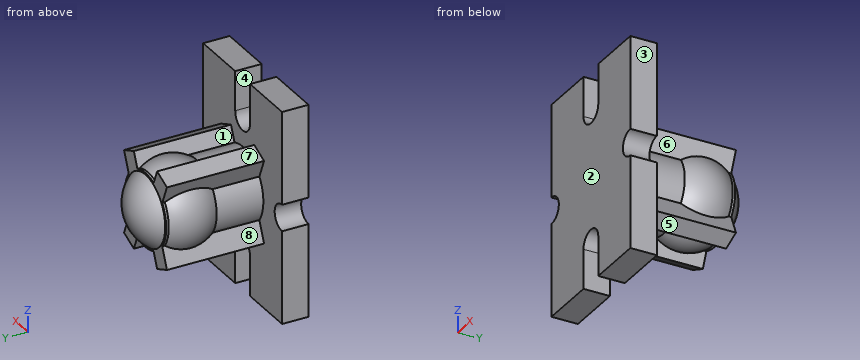
from build123d import *

# Parameters (mm, degrees)
EXTRUDE_1_DEPTH = 3
EXTRUDE_2_DEPTH = 11


with BuildPart() as part:
    # Sketch 1 → Extrude 1 (new body)
    with BuildSketch(Plane(origin=(0, 0, 0), x_dir=(1, 0, 0), z_dir=(0, 1, 0))):
        with BuildLine():
            Line((1.5, 12), (8, 12))
            Line((8, 12), (8, 1.5))
            ThreePointArc((8, 1.5), (6.5, 0), (8, -1.5))
            Line((8, -1.5), (8, -12))
            Line((8, -12), (1.5, -12))
            Line((1.5, -12), (1.5, -7.52))
            ThreePointArc((1.5, -7.52), (0, -6.02), (-1.5, -7.52))
            Line((-1.5, -7.52), (-1.5, -12))
            Line((-1.5, -12), (-8, -12))
            Line((-8, -12), (-8, -1.5))
            ThreePointArc((-8, -1.5), (-6.5, 0), (-8, 1.5))
            Line((-8, 1.5), (-8, 12))
            Line((-8, 12), (-1.5, 12))
            Line((-1.5, 12), (-1.5, 7.52))
            ThreePointArc((-1.5, 7.52), (0, 6.02), (1.5, 7.52))
            Line((1.5, 7.52), (1.5, 12))
        make_face()
    extrude(amount=EXTRUDE_1_DEPTH)



with BuildPart() as body_2:
    # Sketch 2 → Revolve 1 (revolve)
    with BuildSketch(Plane(origin=(0, 0, 0), x_dir=(0, 0, -1), z_dir=(1, 0, 0))):
        with BuildLine():
            Line((0, 16), (0, 6))
            ThreePointArc((0, 6), (5, 11), (0, 16))
        make_face()
    revolve(axis=Axis((0, 3, 0), (0, 1, 0)))


with BuildPart() as part_1:
    add(part.part)

    add(body_2.part)  # Extrude 2 merges body 2
    # Sketch 3 → Extrude 2 (add)
    with BuildSketch(Plane(origin=(0, 3, 0), x_dir=(1, 0, 0), z_dir=(0, 1, 0))):
        with BuildLine():
            Line((1.649838457, 3.862386965), (2.360840268, 5.526891824))
            Line((2.360840268, 5.526891824), (4.347210707, 4.678403474))
            Line((4.347210707, 4.678403474), (3.401303107, 2.46396777))
            ThreePointArc((3.401303107, 2.46396777), (4.2, 0), (3.401303107, -2.46396777))
            Line((3.401303107, -2.46396777), (4.347210707, -4.678403474))
            Line((4.347210707, -4.678403474), (2.360840268, -5.526891824))
            Line((2.360840268, -5.526891824), (1.649838457, -3.862386965))
            ThreePointArc((1.649838457, -3.862386965), (0, -4.2), (-1.649838457, -3.862386965))
            Line((-1.649838457, -3.862386965), (-2.360840268, -5.526891824))
            Line((-2.360840268, -5.526891824), (-4.347210707, -4.678403474))
            Line((-4.347210707, -4.678403474), (-3.401303107, -2.46396777))
            ThreePointArc((-3.401303107, -2.46396777), (-4.2, 0), (-3.401303107, 2.46396777))
            Line((-3.401303107, 2.46396777), (-4.347210707, 4.678403474))
            Line((-4.347210707, 4.678403474), (-2.360840268, 5.526891824))
            Line((-2.360840268, 5.526891824), (-1.649838457, 3.862386965))
            ThreePointArc((-1.649838457, 3.862386965), (0, 4.2), (1.649838457, 3.862386965))
        make_face()
    extrude(amount=EXTRUDE_2_DEPTH)


solid = part_1.part
Input: part model. Units: mm. Frame: model coordinates. Face numbers are marked on the shaded views. A direction names the side the tool comes from. Give positions to 0.01 mm unless a question says otherwise; leave off trailing zeros. Loops run counter-clockwise (first coordinate to the right, second up) from the corner with the lowest first, then second, coordinate; pieces in that order, holes last. Notation, with made-up numbers: M 65.25,75.25 L 86.25,75.25 A24 ccw 86.25,96.25 Z; hole C 2.25,0 d3. An arc over 180 degrees is marked long. Use CSV: the item, a comma, the result in double quotes.
(1) Section C-C, the plane z = 0. Return loops of the section in (x, y), plus the area to 3 significant figures.
Outcome:
outline,"M -6.5,0 L 6.5,0 L 6.5,3 L 4.2,3 L 4.2,8.29 A5 ccw 4.2,13.71 L 4.2,14 L 4,14 A5 ccw -4,14 L -4.2,14 L -4.2,13.71 A5 ccw -4.2,8.29 L -4.2,3 L -6.5,3 Z"
area,"148 mm²"
(2) Material intervals for L1, parallel to X at y = 1.25, z = 9; L2, parallel to Y at x = -5.5, z = -11; L3, parallel to Z at x = -1, y = 11.5, sorted ascending. Write a range as [from, to].
Outcome:
L1,"x = [-8, -1.5], [1.5, 8]"
L2,"y = [0, 3]"
L3,"z = [-4.87, 4.87]"
(3) Section B-B, the plane y = 2.25. Return loops of the section in (x, z), plus the area to 3 significant figures.
Outcome:
outline,"M -8,-12 L -1.5,-12 L -1.5,-7.52 A1.5 cw 1.5,-7.52 L 1.5,-12 L 8,-12 L 8,-1.5 A1.5 cw 8,1.5 L 8,12 L 1.5,12 L 1.5,7.52 A1.5 cw -1.5,7.52 L -1.5,12 L -8,12 L -8,1.5 A1.5 cw -8,-1.5 Z"
area,"343 mm²"
(4) Set-up query: the marked faces 4, 5, 6, 7 and 8. Return all of +Z, -Z, +X, -X, +Y, -Y with unobstructed straight access to the full face (end or side cutting, diameter ignored); none if empty.
Outcome:
face 4,"+Z, +Y, -Y"
face 5,"-Z, +X, +Y"
face 6,"+X"
face 7,"+Z, -X, +Y"
face 8,"-X"
(5) Section A-A, the plane z = -10.5. Return loops of the section in (x, y), plus the area to 3 significant figures.
Outcome:
outline,"M -8,0 L -1.5,0 L -1.5,3 L -8,3 Z; M 1.5,0 L 8,0 L 8,3 L 1.5,3 Z"
area,"39.0 mm²"
(6) Pull-direction query (Y, two-part tool) for the marked faces 1, 2 and 3; classes: pulls with the +Y half, pulls with the -Y half, needs draft (parallel to the pull), parting line crosses it, or undercut.
Outcome:
face 1,"undercut"
face 2,"pulls with the -Y half"
face 3,"needs draft"
(7) Pin query (flat end, axial travel): P1, Ø4, axis at x = 6.5, z = -7, coming from the +Y side; P2, Ø8, axis at y = 11, z = 9, coming from the -X side; P3, Ø8, axis at x = 0.5, y = 12.5, coming from the -Z side. Return the tip coordinate at first contact, or that it passes through.
Outcome:
P1,"stops at y = 3"
P2,"stops at x = -3.59"
P3,"stops at z = -5.53"
(8) Section D-D, the plane y = 6.25. Return loops of the section in (x, z).
Outcome:
outline,"M -4.35,-4.68 L -2.36,-5.53 L -1.65,-3.86 A4.2 ccw 1.65,-3.86 L 2.36,-5.53 L 4.35,-4.68 L 3.4,-2.46 A4.2 ccw 3.4,2.46 L 4.35,4.68 L 2.36,5.53 L 1.65,3.86 A4.2 ccw -1.65,3.86 L -2.36,5.53 L -4.35,4.68 L -3.4,2.46 A4.2 ccw -3.4,-2.46 Z"
